```python
from build123d import *

# Parameters (mm, degrees)
F1_DEPTH  = 15.75
F3_D      = 4
F4_DEPTH  = 3
F5_W      = 3
F5_H      = 15.75
F6_DEPTH  = 25
F8_D      = 2
F9_W      = 6
F9_H      = 4
F10_DEPTH = 15.751
F11_SIZE  = 1
F12_SIZE  = 5
F13_DEPTH = 1
F14_DEPTH = 1
F15_W     = 0.1029567271
F15_H     = 11.4527670667
F15_W_2   = 37.000869453
F16_DEPTH = 15.751
F17_SIZE  = 1.99999


# Not quite as in the source:
# - a fillet or chamfer is up to 0.001 mm smaller than in the source, because OpenCascade refuses the exact size


with BuildPart() as f1:
    # F0 (on Top) → F1 (new body)
    with BuildSketch(Plane.XY):
        Polygon((0, 0), (44.5, 0), (44.5, 10), (37.6, 10), (37.6, 16), (31.6, 16), (31.6, 10), (17.8, 10), (17.8, 16), (11.8, 16), (11.8, 10), (0, 10), align=None)
    extrude(amount=F1_DEPTH)

    # F3 (through all)
    with Locations(Plane.XY.offset(15.75)):
        with Locations((24.7, 5)):
            Hole(F3_D / 2)

    # F4 (add): a face of the model
    f4_faces = [f1.faces().sort_by_distance(p)[0] for p in [
        (0, 5, 7.875),
    ]]
    extrude(f4_faces, amount=F4_DEPTH)

    # F5 (on face) → F6 (join)
    with BuildSketch(Plane(origin=(0, 10, 0), x_dir=(-1, 0, 0), z_dir=(0, 1, 0))):
        with Locations((1.5, 7.875)):
            Rectangle(F5_W, F5_H)
    extrude(amount=F6_DEPTH)

    # F8 (through all)
    with Locations(Plane.YZ):
        with Locations((27.25, 7.875), (17.75, 7.875)):
            Hole(F8_D / 2)

    # F9 (on face) → F10 (cut, through all)
    with BuildSketch(Plane.XY.offset(15.75)):
        with Locations((3, 8)):
            Rectangle(F9_W, F9_H)
    extrude(amount=-F10_DEPTH, mode=Mode.SUBTRACT)

    # F11
    f11_edges = [f1.edges().sort_by_distance(p)[0] for p in [
        (11.8, 16, 7.875),
        (17.8, 16, 7.875),
        (31.6, 16, 7.875),
        (37.6, 16, 7.875),
    ]]
    chamfer(f11_edges, length=F11_SIZE)

    # F12
    f12_edges = [f1.edges().sort_by_distance(p)[0] for p in [
        (44.5, 0, 7.875),
    ]]
    chamfer(f12_edges, length=F12_SIZE)

    # F13 (add): a face of the model
    f13_faces = [f1.faces().sort_by_distance(p)[0] for p in [
        (-3, 0.3838049635, 7.875),
    ]]
    extrude(f13_faces, amount=F13_DEPTH)

    # F14 (cut): a face of the model
    f14_faces = [f1.faces().sort_by_distance(p)[0] for p in [
        (0, 20.4721036707, 7.875),
    ]]
    extrude(f14_faces, amount=-F14_DEPTH, mode=Mode.SUBTRACT)

    # F15 (on face) → F16 (cut, through all)
    with BuildSketch(Plane.XY.offset(15.75)):
        with Locations((5.9485216364, 18.7263835333)):
            Rectangle(F15_W, F15_H)
        Polygon((6, 13), (5.8970432729, 13), (5.8970432729, 24.4527670667), (6, 24.4527670667), (6, 35.557191819), (-12.8509793431, 35.557191819), (-12.8509793431, -2.8801800217), (6, -2.8801800217), (6, 8), align=None)
        with Locations((24.5004347265, 18.7263835333)):
            Rectangle(F15_W_2, F15_H)
        Polygon((49.3548065424, 8), (6, 8), (6, -2.8801800217), (6, -4.4490518048), (49.3548065424, -4.4490518048), align=None)
    extrude(amount=-F16_DEPTH, mode=Mode.SUBTRACT)

    # F17 (size 2 in the source; OpenCascade refuses exactly that, so slightly less here)
    f17_edges = [f1.edges().sort_by_distance(p)[0] for p in [
        (6, 8, 7.875),
        (44.5, 8, 7.875),
    ]]
    chamfer(f17_edges, length=F17_SIZE)


solid = f1.part
```
Read the model definition and answer for the solid it produces. Units are mm, in the model's axes. A direction names the side the tool comes from. Give positions to 0.01 mm unless a question says otherwise; leave off trailing zeros. Order: outer loops, then holes, each group sorted by start corner. A loop starts at its lowest first (then second) coordinate and runs counter-clockwise, first axis right, second up. Notation, with made-up numbers: (72.5, 35.5) -> (118.5, 35.5) arc R24 ccw to (118.5, 52.5) -> close; hole circle Ø2 at (11.5, 20.25). An arc over 180 degrees is marked (long way). Write item = value, one per line.
1. The mould has two halves that part along X. Classify faces 1 (the face through (43.5, 9, 8)), 2 (the face through (17.8, 11, 8)), 3 (the face through (35, 13, 8)), 4 (the face through (31.6, 12, 8)): +X half, -X half, draft (parallel to the pull), parting line (faces both ways), or undercut.
Numbers:
face_1 = +X half
face_2 = undercut
face_3 = draft
face_4 = undercut
2. A cutting plane is placed at A-A, the plane y = 10.85. Write down the section's boundary in (x, z).
Numbers:
outline = (11.8, 0) -> (17.8, 0) -> (17.8, 15.75) -> (11.8, 15.75) -> close; (31.6, 0) -> (37.6, 0) -> (37.6, 15.75) -> (31.6, 15.75) -> close
3. Given pin 1 (1.5 mm diameter, centred on y = 10.5, z = 2.5, fed in from +X); pin 2 (1.5 mm diameter, centred on y = 11.5, z = 6, fed in from -X); pin 3 (1.5 mm diameter, centred on y = 12, z = 9.5, fed in from +X), each flat-ended and moving along its own axis, determine where each tip first touches the part or whether it passes through.
Numbers:
pin_1 = 44.5
pin_2 = 11.8
pin_3 = 37.6
4. Straight lines are drawn through the part: line 1 along X through (y, z) = (12.35, 9.5); line 2 along Y through (x, z) = (30, 7); line 3 along X through (y, z) = (9, 8). For each, find the intervals that lie inside material, in ascending order.
Numbers:
line_1 = 11.8 to 17.8, 31.6 to 37.6
line_2 = 8 to 10
line_3 = 7 to 43.5
5. For faces 5 (the face through (11.8, 12, 8)), 6 (the face through (37.6, 11, 8)), 7 (the face through (25, 10, 8)), determine the directions among +Z, -Z, +X, -X, +Y, -Y from which every point of the face is accessible in a straight line to the end or side of a thin tool.
Numbers:
face_5 = +Z, -Z, -X, +Y
face_6 = +Z, -Z, +X, +Y
face_7 = +Z, -Z, +Y
6. A cutting plane is placed at C-C, the plane x = 22. Write down the section's boundary in (y, z), and give its area (3 significant figures).
Numbers:
outline = (8, 0) -> (10, 0) -> (10, 15.75) -> (8, 15.75) -> close
area = 31.5 mm²
